Geometry: see drawing. Coordinates: mm, zero at the bounding-box minimum. Coordinates: 2 decimals unless noted, no trailing zeros. Loops run counter-clockwise (first coordinate to the right, second up) from the corner with the lowest first, then second, coordinate; pieces in that order, holes last. Notation, with made-up numbers: (82, 42.5) -> (112, 42.5) arc R30 ccw to (112, 67.5) -> close; hole circle Ø11 at (10.5, 76.5). An arc over 180 degrees is marked (long way). Put each result on its own line as item: value. Start each with the question number.
1) Cut plane C-C (y = 222). Return the cut outline in (x, z) (1 decimal).
2) Cut plane B-B (x = 77). Return the cut outline in (y, z).
3) Material intervals for L1, parallel to Y at x = 707.5, z = 4.5; L2, parallel to Y at x = 869, z = 9.25, sorted ascending.
4) Contact query for a flat-ended pin moving along its axis: P1, Ø3, axis at x = 785, z = 5.5, coming from the -Y side. Output: stop coordinate, or through.
5) Cut plane A-A (z = 7.5). Return the cut outline in (x, y).
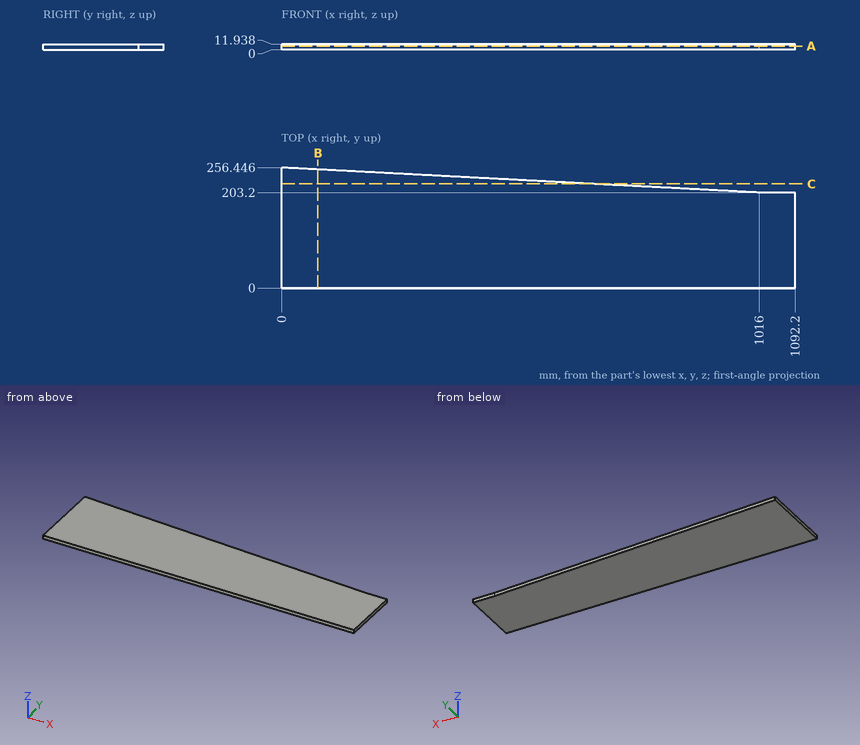
Results found:
1. outline: (0, 0) -> (657.3, 0) -> (657.3, 11.9) -> (0, 11.9) -> close
2. outline: (0, 0) -> (252.41, 0) -> (252.41, 11.94) -> (0, 11.94) -> close
3. L1: y = 0 to 219.37
3. L2: y = 0 to 210.9
4. P1: stops at y = 0
5. outline: (0, 0) -> (1092.2, 0) -> (1092.2, 203.2) -> (1016, 203.2) -> (0, 256.45) -> close
